CAD build for the part. Positions are in the model's coordinates, mm. Coordinates: 2 decimals unless noted, no trailing zeros. Loops run counter-clockwise (first coordinate to the right, second up) from the corner with the lowest first, then second, coordinate; pieces in that order, holes last. Notation, with made-up numbers: (77.5, 13.25) -> (92.5, 13.25) arc R11 ccw to (92.5, 23.25) -> close; hole circle Ø5 at (-31.75, -15). An arc over 180 degrees is marked (long way). Return JSON: item names as keys, results as strings. Group by question number.
(1) Saw through at B-B on z = 1.6. Give the number of separate pieces and of enclosed holes in the cut face, then the cut area to 3 significant figures.
(2) Probe L1, parallel to Y at x = -30, z = 5.65; L2, parallel to Y at x = 9, z = 4.8; L3, parallel to X at y = -17.5, z = 3.6. List the from-to ranges inside material, lowest first.
(3) Saw through at A-A on y = 9.85. Write the cut outline in (x, z).
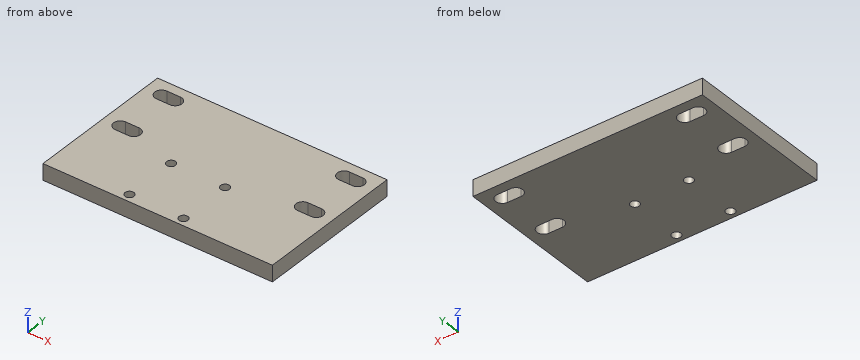
```python
from build123d import *

# Parameters (mm, degrees)
SKETCH2_W           = 85
SKETCH2_H           = 55.083692651
SKETCH2_R           = 1.65
BOSS_EXTRUDE1_DEPTH = 6


with BuildPart() as part:
    # Sketch2 → Boss-Extrude1 (new body)
    with BuildSketch(Plane.XY):
        with Locations((2.5, -11.594499981)):
            Rectangle(SKETCH2_W, SKETCH2_H)
        with Locations((-10.268789461, -16.131613602)):
            Circle(SKETCH2_R, mode=Mode.SUBTRACT)
        with Locations((9.731210539, -16.131613602)):
            Circle(SKETCH2_R, mode=Mode.SUBTRACT)
        with Locations((-10.268789461, -36.131613602)):
            Circle(SKETCH2_R, mode=Mode.SUBTRACT)
        with Locations((9.747732282, -36.131613602)):
            Circle(SKETCH2_R, mode=Mode.SUBTRACT)
        with BuildLine():
            Line((-33.8, 12.35), (-28.8, 12.35))
            ThreePointArc((-28.8, 12.35), (-26.3, 9.85), (-28.8, 7.35))
            Line((-28.8, 7.35), (-33.8, 7.35))
            ThreePointArc((-33.8, 7.35), (-36.3, 9.85), (-33.8, 12.35))
        make_face(mode=Mode.SUBTRACT)
        with BuildLine():
            Line((-33.8, -7.5), (-28.8, -7.5))
            ThreePointArc((-28.8, -7.5), (-26.3, -10), (-28.8, -12.5))
            Line((-28.8, -12.5), (-33.8, -12.5))
            ThreePointArc((-33.8, -12.5), (-36.3, -10), (-33.8, -7.5))
        make_face(mode=Mode.SUBTRACT)
        with BuildLine():
            Line((38.8, 12.35), (33.8, 12.35))
            ThreePointArc((33.8, 12.35), (31.3, 9.85), (33.8, 7.35))
            Line((33.8, 7.35), (38.8, 7.35))
            ThreePointArc((38.8, 7.35), (41.3, 9.85), (38.8, 12.35))
        make_face(mode=Mode.SUBTRACT)
        with BuildLine():
            Line((38.8, -7.5), (33.8, -7.5))
            ThreePointArc((33.8, -7.5), (31.3, -10), (33.8, -12.5))
            Line((33.8, -12.5), (38.8, -12.5))
            ThreePointArc((38.8, -12.5), (41.3, -10), (38.8, -7.5))
        make_face(mode=Mode.SUBTRACT)
    extrude(amount=BOSS_EXTRUDE1_DEPTH)


solid = part.part
```
Geometry results:
{
 "1": {"separate pieces": "1", "enclosed holes": "8", "area": "4,470 mm²"},
 "2": {"L1": "-39.14 to -12.5, -7.5 to 7.35, 12.35 to 15.95", "L2": "-39.14 to -37.6, -34.66 to -17.61, -14.65 to 15.95", "L3": "-40 to -11.19, -9.35 to 8.81, 10.65 to 45"},
 "3": {"outline": "(-40, 0) -> (-36.3, 0) -> (-36.3, 6) -> (-40, 6) -> close; (-26.3, 0) -> (31.3, 0) -> (31.3, 6) -> (-26.3, 6) -> close; (41.3, 0) -> (45, 0) -> (45, 6) -> (41.3, 6) -> close"}
}
